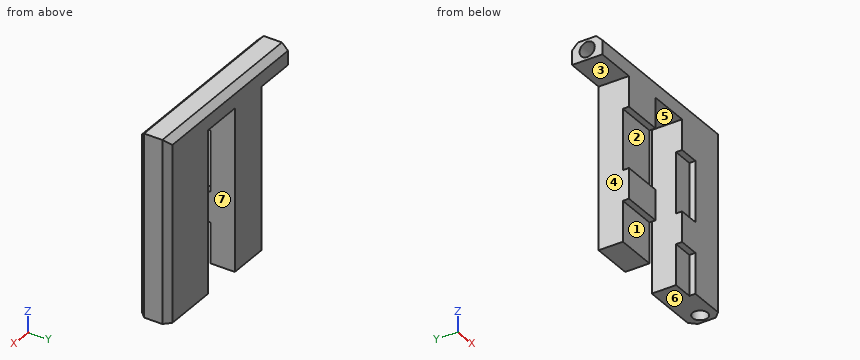
```python
from build123d import *

# Parameters (mm, degrees)
SKETCH1_W           = 50.8
SKETCH1_H           = 203.2
BOSS_EXTRUDE1_DEPTH = 38.1
SKETCH3_R           = 9.525
CUT_EXTRUDE1_DEPTH  = 38.1
SKETCH4_R           = 9.525
CUT_EXTRUDE2_DEPTH  = 38.1
CUT_EXTRUDE3_DEPTH  = 7.62
SKETCH6_W           = 127
SKETCH6_H           = 76.2
CUT_EXTRUDE4_DEPTH  = 7.62
CHAMFER1_SIZE       = 7.62


with BuildPart() as part:
    # Sketch1 → Boss-Extrude1 (new body)
    with BuildSketch(Plane(origin=(0, 0, 0), x_dir=(1, 0, 0), z_dir=(0, 1, 0))):
        Polygon((-25.4, 228.6), (-25.4, 25.4), (-76.2, 25.4), (-127, 25.4), (-177.8, 25.4), (-228.6, 25.4), (-228.6, 0), (0, 0), (0, 228.6), align=None)
        with Locations((-50.8, 127)):
            Rectangle(SKETCH1_W, SKETCH1_H)
        with Locations((-152.4, 127)):
            Rectangle(SKETCH1_W, SKETCH1_H)
    extrude(amount=BOSS_EXTRUDE1_DEPTH)

    # Sketch3 → Cut-Extrude1 (cut)
    with BuildSketch(Plane.ZY.offset(228.6)):
        with Locations((-12.7, 19.05)):
            Circle(SKETCH3_R)
    extrude(amount=-CUT_EXTRUDE1_DEPTH, mode=Mode.SUBTRACT)

    # Sketch4 → Cut-Extrude2 (cut)
    with BuildSketch(Plane(origin=(0, 0, -228.6), x_dir=(-1, 0, 0), z_dir=(0, 0, -1))):
        with Locations((12.684892179, 19.05)):
            Circle(SKETCH4_R)
    extrude(amount=-CUT_EXTRUDE2_DEPTH, mode=Mode.SUBTRACT)

    # Sketch5 → Cut-Extrude3 (cut)
    with BuildSketch(Plane(origin=(0, 0, 0), x_dir=(-1, 0, 0), z_dir=(0, -1, 0))):
        Polygon((50.8, 431.742057994), (50.8, 177.742057994), (279.4, 177.742057994), (279.4, 431.771028997), align=None)
    extrude(amount=-CUT_EXTRUDE3_DEPTH, mode=Mode.SUBTRACT)

    # Sketch6 → Cut-Extrude4 (cut)
    with BuildSketch(Plane(origin=(0, 0, 0), x_dir=(-1, 0, 0), z_dir=(0, -1, 0))):
        with Locations((114.3, 101.571028997)):
            Rectangle(SKETCH6_W, SKETCH6_H)
    extrude(amount=-CUT_EXTRUDE4_DEPTH, mode=Mode.SUBTRACT)

    # Chamfer1
    chamfer1_edges = [part.edges().sort_by_distance(p)[0] for p in [
        (0, 0, -114.3),
        (-114.3, 0, 0),
        (-114.3, 38.1, 0),
        (0, 38.1, -114.3),
    ]]
    chamfer(chamfer1_edges, length=CHAMFER1_SIZE)


solid = part.part
```
Verification items for the finished model (mm, model axes). Face numbers are marked on the shaded views. A direction names the side the tool comes from. Give positions to 0.01 mm unless a question says otherwise; leave off trailing zeros. Loops run counter-clockwise (first coordinate to the right, second up) from the corner with the lowest first, then second, coordinate; pieces in that order, holes last. Notation, with made-up numbers: M 24.25,2.5 L 50.25,2.5 A21 cw 50.25,15.5 Z; hole C 53,42 d9. An arc over 180 degrees is marked long. Return JSON: item names as keys, results as strings.
1) Mould release check, pull along X, two halves, no side actions. Record for the marked faces 4, 5, 6 and 7: released by +X, released by -X, zero draft, split by the parting line, or undercut.
Findings:
{"face 4": "released by -X", "face 5": "undercut", "face 6": "zero draft", "face 7": "undercut"}
2) Gauge pin test, flat ends, axial feed: P1, Ø9.5, axis at x = -12, y = 16.5, coming from the -Z side; P2, Ø11.5, axis at x = -93, y = 25, coming from the -Z side; P3, Ø4, axis at x = -148.5, y = 2, coming from the -Z side. Record the tip position at first contact, or that the pin passes through.
Findings:
{"P1": "stops at z = -190.5", "P2": "stops at z = -25.4", "P3": "stops at z = -177.74"}
3) Material ranges on L1, parallel to X at y = 18, z = -201; L2, parallel to Y at x = -209, z = -12; L3, parallel to X at y = 9.5, z = -82.5, recorded low to high. Write a range as [from, to].
Findings:
{"L1": "x = [-177.8, -127], [-76.2, -22.15], [-3.22, 0]", "L2": "y = [0, 9.55], [28.55, 38.1]", "L3": "x = [-177.8, -127], [-76.2, 0]"}
4) Section check B-B, the plane x = -65. Enter the section's corners in (y, z), and give its area (3 significant figures).
Findings:
{"outline": "M 0,-177.74 L 7.62,-177.74 L 7.62,-228.6 L 38.1,-228.6 L 38.1,-7.62 L 30.48,0 L 7.62,0 L 0,-7.62 L 0,-63.47 L 7.62,-63.47 L 7.62,-139.67 L 0,-139.67 Z", "area": "7,680 mm2"}
5) Section check D-D, the plane z = -155.5. Enter the section's corners in (x, y).
Findings:
{"outline": "M -177.8,0 L -127,0 L -127,38.1 L -177.8,38.1 Z; M -76.2,0 L -7.62,0 L 0,7.62 L 0,30.48 L -7.62,38.1 L -76.2,38.1 Z"}
6) Section check C-C, the plane y = 19.05. Enter the section's corners in (x, z) (3 decimals), and give its area (3 significant figures).
Findings:
{"outline": "M -228.6,-25.4 L -177.8,-25.4 L -177.8,-228.6 L -127,-228.6 L -127,-25.4 L -76.2,-25.4 L -76.2,-228.6 L -22.21,-228.6 L -22.21,-190.5 L -3.16,-190.5 L -3.16,-228.6 L 0,-228.6 L 0,0 L -228.6,0 L -228.6,-3.175 L -190.5,-3.175 L -190.5,-22.225 L -228.6,-22.225 Z", "area": "30,200 mm2"}
7) Tool access check on the marked faces 1, 2 and 3. Record the directions out of +Z, -Z, +X, -X, +Y, -Y that give a thin tool (end or side, any length) a straight path to the whole face; none if there is none.
Findings:
{"face 1": "-Z, -X, -Y", "face 2": "-X, -Y", "face 3": "-Z, -X, +Y, -Y"}
8) Section check A-A, the plane z = -115. Enter the section's corners in (x, y).
Findings:
{"outline": "M -177.8,7.62 L -127,7.62 L -127,38.1 L -177.8,38.1 Z; M -76.2,7.62 L -50.8,7.62 L -50.8,0 L -7.62,0 L 0,7.62 L 0,30.48 L -7.62,38.1 L -76.2,38.1 Z"}
